The listing builds one solid part. Answer for the finished solid, in the listing's coordinates (mm). A direction names the side the tool comes from. Coordinates: 2 decimals unless noted, no trailing zeros. Order: outer loops, then holes, each group sorted by start corner. A loop starts at its lowest first (then second) coordinate and runs counter-clockwise, first axis right, second up. Notation, with made-up numbers: (52, -24) - (70, -24) arc R8 ccw to (70, -19) - close; hole circle Ø9 at (51, -34.75). An arc over 180 degrees is marked (long way). Use a Markdown table: item, result. Add a question column.
Item 1: The mould has two halves that part along Y. Classify faces 1 (the flat face through (397, 29, -15)), 2 (the flat face through (-6, 2, -15)), 3 (the flat face through (-6, 0, -15)): released by +Y, released by -Y, zero draft, split by the parting line, or undercut.
Item 2: Find the intervals of material crossed by line 1 along Z through (x, y) = (358, 5.5); line 2 along Z through (x, y) = (343, 3.25); line 3 along Y through (x, z) = (274, -22), in increasing order.
Item 3: The part is cut by section C-C, the plane x = -222.5. Give the vertices of the cut face in (y, z), then the cut area to 3 significant figures.
Item 4: The part is cut by section A-A, the plane y = 21.5. Give the vertices of the cut face in (x, z).
Item 5: The part is cut by section B-B, the plane z = -11.75. Give the vertices of the cut face in (x, y), then the cut area to 3 significant figures.
Item 6: For faces 4 (the flat face through (-6, 28, -15)), 5 (the flat face through (-6, 15, 0)), determine the directions among +Z, -Z, +X, -X, +Y, -Y from which every point of the face is accessible in a straight line to the end or side of a thin tool.
from build123d import *

# Parameters (mm, degrees)
EXTRUDE_1_DEPTH = 397


with BuildPart() as part:
    # Эскиз1 → Бобышка-Вытянуть1 (new body)
    with BuildSketch(Plane(origin=(0, 0, 0), x_dir=(0, 0, -1), z_dir=(1, 0, 0))):
        with BuildLine():
            Line((3, 30), (27, 30))
            ThreePointArc((27, 30), (29.121320344, 29.121320344), (30, 27))
            Line((30, 27), (30, 3))
            ThreePointArc((30, 3), (29.121320344, 0.878679656), (27, 0))
            Line((27, 0), (3, 0))
            ThreePointArc((3, 0), (0.878679656, 0.878679656), (0, 3))
            Line((0, 3), (0, 27))
            ThreePointArc((0, 27), (0.878679656, 29.121320344), (3, 30))
        make_face()
        with BuildLine():
            Line((4, 28), (26, 28))
            ThreePointArc((26, 28), (27.414213562, 27.414213562), (28, 26))
            Line((28, 26), (28, 4))
            ThreePointArc((28, 4), (27.414213562, 2.585786438), (26, 2))
            Line((26, 2), (4, 2))
            ThreePointArc((4, 2), (2.585786438, 2.585786438), (2, 4))
            Line((2, 4), (2, 26))
            ThreePointArc((2, 26), (2.585786438, 27.414213562), (4, 28))
        make_face(mode=Mode.SUBTRACT)
    extrude(amount=-EXTRUDE_1_DEPTH)

    # Зеркальное отражение2: part across plane


with BuildPart() as part_1:
    add(part.part)
    add(part.part.mirror(Plane(origin=(0, 3, -3), x_dir=(0, 0, 1), z_dir=(1, 0, 0))))


solid = part_1.part
Solution:
| question | item | result |
|---|---|---|
| 1 | face 1 | zero draft |
| 1 | face 2 | undercut |
| 1 | face 3 | released by -Y |
| 2 | line 1 | z = -30 to -28, -2 to 0 |
| 2 | line 2 | z = -30 to -27.85, -2.15 to 0 |
| 2 | line 3 | y = 0 to 2, 28 to 30 |
| 3 | outline | (0, -27) arc R3 ccw to (3, -30) - (27, -30) arc R3 ccw to (30, -27) - (30, -3) arc R3 ccw to (27, 0) - (3, 0) arc R3 ccw to (0, -3) - close; hole (2, -26) arc R2 ccw to (4, -28) - (26, -28) arc R2 ccw to (28, -26) - (28, -4) arc R2 ccw to (26, -2) - (4, -2) arc R2 ccw to (2, -4) - close |
| 3 | area | 220 mm2 |
| 4 | outline | (-397, -30) - (397, -30) - (397, -28) - (-397, -28) - close; (-397, -2) - (397, -2) - (397, 0) - (-397, 0) - close |
| 5 | outline | (-397, 0) - (397, 0) - (397, 2) - (-397, 2) - close; (-397, 28) - (397, 28) - (397, 30) - (-397, 30) - close |
| 5 | area | 3,180 mm2 |
| 6 | face 4 | +X, -X |
| 6 | face 5 | +Z, +X, -X, +Y, -Y |
